Read the model definition and answer for the solid it produces. Units are mm, in the model's axes. A direction names the side the tool comes from. Coordinates: 2 decimals unless noted, no trailing zeros. Loops run counter-clockwise (first coordinate to the right, second up) from the corner with the lowest first, then second, coordinate; pieces in that order, holes last.
from build123d import *

# Parameters (mm, degrees)
F0_R     = 11.1
F1_DEPTH = 1.2
F0_R_2   = 12.85
F2_DEPTH = 60
F3_W     = 62.815846
F3_H     = 60.049228
F4_DEPTH = 3


with BuildPart() as f1:
    # F0 (on Top) → F1 (new body)
    with BuildSketch(Plane.XY):
        Circle(F0_R)
    extrude(amount=F1_DEPTH)

    # F0 (on Top) → F2 (join)
    with BuildSketch(Plane.XY):
        Circle(F0_R_2)
        Circle(F0_R, mode=Mode.SUBTRACT)
    extrude(amount=F2_DEPTH)

    # F3 (on Front) → F4 (join)
    with BuildSketch(Plane.XZ):
        with Locations((0, 30.024614)):
            Rectangle(F3_W, F3_H)
    extrude(amount=F4_DEPTH)


solid = f1.part
Item 1: A cutting plane is placed at C-C on y = 7.5. Determine the outline of the cut face in (x, z), then the cut area to 3 significant figures.
Numbers:
outline: (-10.43, 0) - (10.43, 0) - (10.43, 60) - (8.18, 60) - (8.18, 1.2) - (-8.18, 1.2) - (-8.18, 60) - (-10.43, 60) - close
area: 290 mm2
Item 2: Which of the six approach directions +Z, -Z, +X, -X, +Y, -Y give full straight-line access (tool end or side, diameter ignored) to faces 1 (the face through (0, 0, 30)), 2 (the face through (0, -2, 0))?
Numbers:
face 1: +Z
face 2: -Z, +X, -X, +Y, -Y
Item 3: Determine the mould class of faces 3 (the face through (0.283, 12.847, 29.58)), 4 (the face through (-31.408, -1, 30)), 5 (the face through (-0.24, -12.848, 29.58)), 6 (the face through (0, -6, 1.2)) for opening direction Y: released by +Y, released by -Y, zero draft, split by the parting line, or undercut.
Numbers:
face 3: released by +Y
face 4: zero draft
face 5: released by -Y
face 6: undercut
Item 4: A cutting plane is placed at D-D on x = -25. Determine the outline of the cut face in (y, z).
Numbers:
outline: (-3, 0) - (0, 0) - (0, 60.05) - (-3, 60.05) - close
Item 5: A cutting plane is placed at A-A on z = 6.5. Determine the outline of the cut face in (x, y).
Numbers:
outline: (-31.41, -3) - (-12.49, -3) arc R12.85 ccw to (12.49, -3) - (31.41, -3) - (31.41, 0) - (12.85, 0) arc R12.85 ccw to (-12.85, 0) - (-31.41, 0) - close; hole (-11.1, 0) - (11.1, 0) arc R11.1 ccw to start; hole (-10.69, -3) arc R11.1 ccw to (10.69, -3) - close
Item 6: Find the intervals of material crossed by line 1 along Y through (x, z) = (3.5, 7); line 2 along X through (y, z) = (0.25, 39.5); line 3 along Y through (x, z) = (24, 57.5), in increasing order.
Numbers:
line 1: y = -12.36 to -10.53, -3 to 0, 10.53 to 12.36
line 2: x = -12.85 to -11.1, 11.1 to 12.85
line 3: y = -3 to 0
Item 7: A cutting plane is placed at B-B on x = 0. Determine the outline of the cut face in (y, z).
Numbers:
outline: (-12.85, 0) - (12.85, 0) - (12.85, 60) - (11.1, 60) - (11.1, 1.2) - (0, 1.2) - (0, 60.05) - (-3, 60.05) - (-3, 1.2) - (-11.1, 1.2) - (-11.1, 60) - (-12.85, 60) - close
Item 8: Given pin 1 (5 mm diameter, centred on x = -2.5, y = -8, fed in from +Z); pin 2 (12 mm diameter, centred on y = 9, z = 21.5, fed in from -X); pin 3 (12 mm diameter, centred on x = -11.5, z = 11, fed in from -Y); pin 4 (12 mm diameter, centred on x = 23, y = -9.5, fed in from -Z), each flat-ended and moving along its own axis, determine where each tip first touches the part or whether it passes through.
Numbers:
pin 1: stops at z = 1.2
pin 2: stops at x = -12.49
pin 3: stops at y = -11.61
pin 4: passes through
